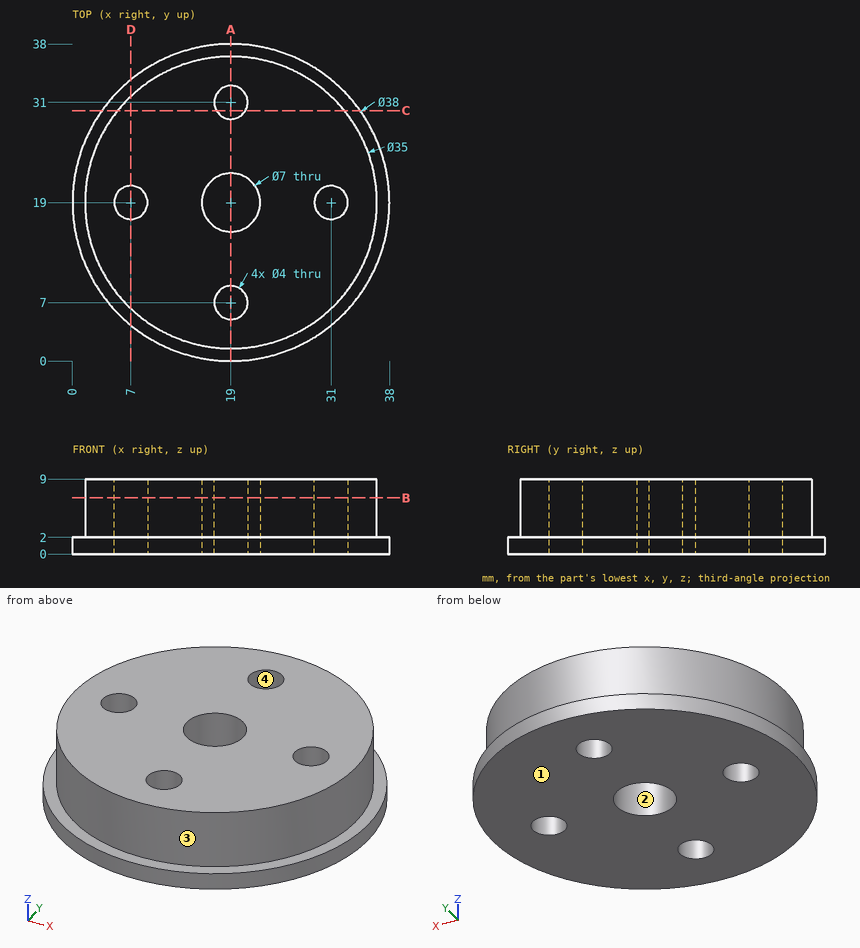
Geometry check sheet. Reference: drawing and pictorial views, mm from the part's lowest x, y, z. Give positions to 0.01 mm unless a question says otherwise; leave off trailing zeros. Loops run counter-clockwise (first coordinate to the right, second up) from the corner with the lowest first, then second, coordinate; pieces in that order, holes last. Notation, with made-up numbers: (28, 55.25) - (69, 55.25) arc R19 cw to (69, 82.25) - close; hole circle Ø10 at (88.5, 63.25). An arc over 180 degrees is marked (long way). One line per question, with ' | ' between items. Start each with the question number.
1. Cross-section at D-D, the plane x = 7. Enter the section's corners in (y, z), plus the area to 3 significant figures.
2. Material ranges on line 1 along Y through (x, z) = (19, 4.75); line 2 along Y through (x, z) = (19.5, 6.75); line 3 along X through (y, z) = (8, 2.25), recorded low to high. Write a range as [from, to].
3. Draft check along X on the marked faces 1, 2, 3 and 4. Enter one of: released by +X, released by -X, zero draft, split by the parting line, or undercut.
4. Cross-section at C-C, the plane y = 30. Enter the section's corners in (x, z), plus the area to 3 significant figures.
5. Cross-section at B-B, the plane z = 6.75. Enter the section's corners in (x, y).
6. Cross-section at A-A, the plane x = 19. Enter the section's corners in (y, z).
7. Gauge pin test, flat ends, axial feed: pin 1 Ø3 at (y, z) = (6, 1.5) entering from +X; pin 2 Ø1.5 at (x, z) = (30.5, 7.5) entering from -Y; pin 3 Ø3 at (x, z) = (32, 4.5) entering from -Y. Record the tip position at first contact, or that the pin passes through.
Check result:
1) outline: (4.27, 0) - (17, 0) - (17, 9) - (6.26, 9) - (6.26, 2) - (4.27, 2) - close; (21, 0) - (33.73, 0) - (33.73, 2) - (31.74, 2) - (31.74, 9) - (21, 9) - close | area: 201 mm2
2) line 1: y = [1.5, 5], [9, 15.5], [22.5, 29], [33, 36.5] | line 2: y = [1.51, 5.06], [8.94, 15.54], [22.46, 29.06], [32.94, 36.49] | line 3: x = [5.39, 17.27], [20.73, 32.61]
3) face 1: zero draft | face 2: undercut | face 3: split by the parting line | face 4: undercut
4) outline: (3.51, 0) - (17.27, 0) - (17.27, 9) - (5.39, 9) - (5.39, 2) - (3.51, 2) - close; (20.73, 0) - (34.49, 0) - (34.49, 2) - (32.61, 2) - (32.61, 9) - (20.73, 9) - close | area: 221 mm2
5) outline: circle Ø35 at (19, 19); hole circle Ø4 at (7, 19); hole circle Ø7 at (19, 19); hole circle Ø4 at (19, 7); hole circle Ø4 at (19, 31); hole circle Ø4 at (31, 19)
6) outline: (0, 0) - (5, 0) - (5, 9) - (1.5, 9) - (1.5, 2) - (0, 2) - close; (9, 0) - (15.5, 0) - (15.5, 9) - (9, 9) - close; (22.5, 0) - (29, 0) - (29, 9) - (22.5, 9) - close; (33, 0) - (38, 0) - (38, 2) - (36.5, 2) - (36.5, 9) - (33, 9) - close
7) pin 1: stops at x = 34.12 | pin 2: stops at y = 5.19 | pin 3: stops at y = 5.81
